Part print with two shaded views. Sizes in mm from the minimum x, y, z corner. A direction names the side the tool comes from. Round coordinates to 2 decimals unless told otherwise and drop trailing zeros. Loops run counter-clockwise (first coordinate to the right, second up) from the corner with the lowest first, then second, coordinate; pieces in that order, holes last. Notation, with made-up numbers: M 19.25,14.5 L 56.25,14.5 A25 ccw 56.25,46.5 Z; hole C 26,28.25 d1. An arc over 180 degrees is marked long. Answer as CSV lines item,"result". Start each with the question number.
Item 1: Which spindle directions (+Z, -Z, +X, -X, +Y, -Y) get a long thin tool onto all of the face, cutting with end or side? Do the marked faces 1, 2 and 3. Say none if no direction does.
Item 2: Wall check: line 1 (X direction, y = 4.5, z = 18) (1 decimal); line 2 (X direction, y = 17.5, z = 24) (1 decimal); line 3 (X direction, y = 27, z = 1.75). Give the ranges that are in metal, low to high.
Item 3: Band-saw the part on C-C (x = 12). Give the cut face in (y, z).
Item 4: Mould opens along X. For the marked faces 4, 5, 6 and 7 say: pulls with the +X half, pulls with the -X half, needs draft (parallel to the pull), parting line crosses it, or undercut.
Item 5: Drop flat-ended pins along their axis: pin 1 Ø3 at (y, z) = (4.5, 19.5) entering from -X (3 decimals); pin 2 Ø5 at (y, z) = (30.5, 12) entering from +X (3 decimals); pin 3 Ø8 at (x, z) = (54.5, 11.5) entering from +Y. Give the stop position or say it passes through.
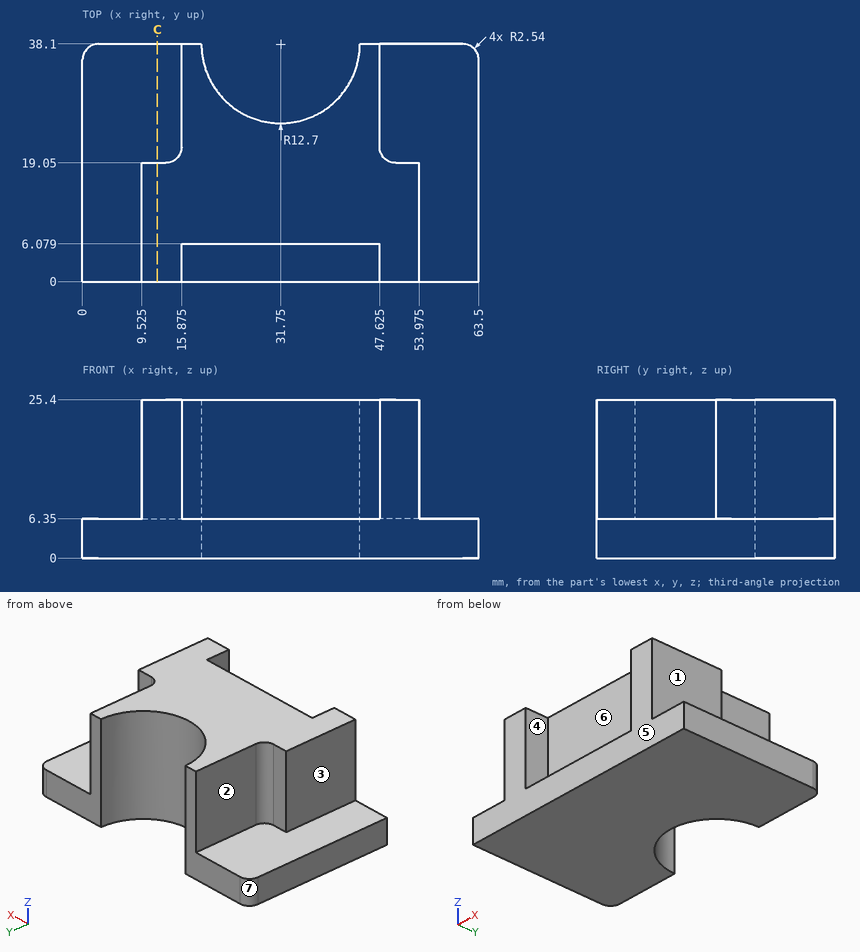
Answer block:
1,face 1,"+Z, +X, +Y, -Y"
1,face 2,"+Z, -X, +Y"
1,face 3,"+Z, -X, +Y, -Y"
2,line 1,"x = 9.5 to 15.9, 47.6 to 54"
2,line 2,"x = 9.5 to 54"
2,line 3,"x = 0 to 25.58, 37.92 to 63.5"
3,outline,"M 0,0 L 38.1,0 L 38.1,6.35 L 19.05,6.35 L 19.05,25.4 L 0,25.4 Z"
4,face 4,"undercut"
4,face 5,"needs draft"
4,face 6,"undercut"
4,face 7,"pulls with the -X half"
5,pin 1,"stops at x = 9.525"
5,pin 2,"stops at x = 47.625"
5,pin 3,"stops at y = 19.05"
